from build123d import *

# Parameters (mm, degrees)
F0_W     = 177.8
F0_H     = 127
F1_DEPTH = 76.2
F2_R     = 12.7
F4_DEPTH = 101.6
F6_DEPTH = 50.8
F8_DEPTH = 50.8
F9_R     = 5.08
F10_R    = 5.08


with BuildPart() as f1:
    # F0 (on Top) → F1 (new body)
    with BuildSketch(Plane.XY):
        with Locations((-8.271977, -2.472461)):
            Rectangle(F0_W, F0_H)
        with BuildLine():
            Line((-83.807927, -45.345337), (-83.807927, 28.44747))
            ThreePointArc((-83.807927, 28.44747), (-70.589135, 37.835685), (-57.370342, 28.44747))
            Line((-57.370342, 28.44747), (-57.370342, -45.345337))
            ThreePointArc((-57.370342, -45.345337), (-70.589135, -54.660871), (-83.807927, -45.345337))
        make_face(mode=Mode.SUBTRACT)
        with BuildLine():
            ThreePointArc((38.502203, 28.44747), (51.139944, 41.085211), (63.777684, 28.44747))
            Line((63.777684, 28.44747), (63.777684, -45.345337))
            ThreePointArc((63.777684, -45.345337), (51.139944, -57.983078), (38.502203, -45.345337))
            Line((38.502203, -45.345337), (38.502203, 28.44747))
        make_face(mode=Mode.SUBTRACT)
    extrude(amount=F1_DEPTH)

    # F2
    f2_edges = [f1.edges().sort_by_distance(p)[0] for p in [
        (80.628023, 61.027539, 38.1),
        (80.628023, -65.972461, 38.1),
        (-97.171977, 61.027539, 38.1),
        (-97.171977, -65.972461, 38.1),
    ]]
    fillet(f2_edges, radius=F2_R)

    # F3 (on face) → F4 (join)
    with BuildSketch(Plane.XY.offset(76.2)):
        with BuildLine():
            ThreePointArc((0.43315, 40.995162), (-7.205375, 48.633687), (-14.8439, 40.995162))
            Line((-14.8439, 40.995162), (-14.8439, 15.583021))
            Line((-14.8439, 15.583021), (-41.930374, 15.583021))
            ThreePointArc((-41.930374, 15.583021), (-49.721884, 7.79151), (-41.930374, 0))
            Line((-41.930374, 0), (-14.8439, 0))
            Line((-14.8439, 0), (-14.8439, -28.666684))
            ThreePointArc((-14.8439, -28.666684), (-7.42195, -36.088634), (0, -28.666684))
            Line((0, -28.666684), (0, 0))
            Line((0, 0), (25.956901, 0))
            ThreePointArc((25.956901, 0), (33.748411, 7.79151), (25.956901, 15.583021))
            Line((25.956901, 15.583021), (0.43315, 15.583021))
            Line((0.43315, 15.583021), (0.43315, 40.995162))
        make_face()
    extrude(amount=F4_DEPTH)

    # F5 (on face) → F6 (join)
    with BuildSketch(Plane.YZ):
        Polygon((-16.809505, 118.773863), (-10.288356, 118.773863), (-7.027781, 124.421343), (-10.288356, 130.068824), (-16.809505, 130.068824), (-20.070079, 124.421343), align=None)
    extrude(amount=F6_DEPTH)

    # F7 (on face) → F8 (join)
    with BuildSketch(Plane(origin=(-14.8439, 0, 0), x_dir=(0, -1, 0), z_dir=(-1, 0, 0))):
        Polygon((15.825561, 128.772154), (10.70182, 128.772154), (8.139949, 124.334864), (10.70182, 119.897574), (15.825561, 119.897574), (18.387432, 124.334864), align=None)
    extrude(amount=F8_DEPTH)

    # F9
    f9_edges = [f1.edges().sort_by_distance(p)[0] for p in [
        (0.43315, 28.289091, 177.8),
        (-7.205375, 48.633687, 177.8),
        (-14.8439, 28.289091, 177.8),
        (-28.387137, 15.583021, 177.8),
        (-49.721884, 7.79151, 177.8),
        (-28.387137, 0, 177.8),
        (-14.8439, -14.333342, 177.8),
        (-7.42195, -36.088634, 177.8),
        (0, -14.333342, 177.8),
        (12.97845, 0, 177.8),
        (33.748411, 7.79151, 177.8),
        (13.195026, 15.583021, 177.8),
    ]]
    fillet(f9_edges, radius=F9_R)

    # F10
    f10_edges = [f1.edges().sort_by_distance(p)[0] for p in [
        (-97.171977, -2.472461, 0),
        (-97.171977, 48.327539, 38.1),
        (-97.171977, -53.272461, 38.1),
        (-97.171977, -2.472461, 76.2),
    ]]
    fillet(f10_edges, radius=F10_R)


solid = f1.part
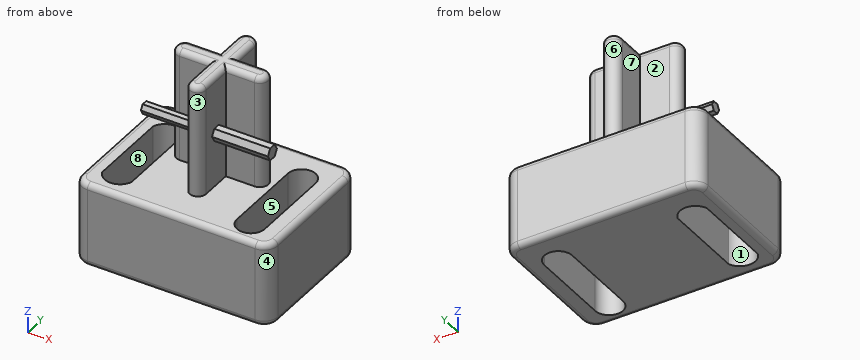
Here's how the part is built. I have some questions about the finished solid (model axes, mm). Face numbers are marked on the shaded views. A direction names the side the tool comes from. Round coordinates to 2 decimals unless told otherwise and drop trailing zeros. Order: outer loops, then holes, each group sorted by start corner. A loop starts at its lowest first (then second) coordinate and runs counter-clockwise, first axis right, second up. Notation, with made-up numbers: M 54.25,55.5 L 106.25,55.5 A29 cw 106.25,90.5 Z; hole C 32,-2.5 d7. An arc over 180 degrees is marked long. Return JSON: item names as keys, results as strings. Group by question number.
1. If we section it at C-C on z = 47: List the corners of the cut face in (x, y) for me, then the cut area to 3 significant figures.
2. If we mould it in two halves opening along X, with no side actions, what happens to the marked faces 1, 2, 3 and 4? For each: pulls with the +X half, pulls with the -X half, needs draft (parallel to the pull), parting line crosses it, or undercut.
3. Please list where these lines run through material, in increasing order: probe 1 along X at (y, z) = (24.5, 17); probe 2 along X at (y, z) = (34.5, 41.5); probe 3 along Z at (x, y) = (-42.5, -35).
4. If we section it at A-A on y = -43: List the corners of the cut face in (x, z) for me.
5. If we section it at B-B on x = -28: List the corners of the cut face in (y, z) for me, then the cut area to 3 significant figures.
6. If we section it at D-D on z = 156.5: List the corners of the cut face in (x, y) for me, then the cut area to 3 significant figures.
7. On a 3-axis mill with a long thin cutter (end or side, diameter ignored), from which of +Z, -Z, +X, -X, +Y, -Y can I reach the whole of each face in a straight line? I mean the marked faces 5, 6, 7 and 8. Say none if no direction works.
8. I'm going to push flat-ended pins straight in: pin 1 Ø6 at (x, z) = (-26.5, 106.5) entering from +Y; pin 2 Ø1.5 at (x, y) = (-58, -16) entering from +Z; pin 3 Ø5 at (x, y) = (32, -12.5) entering from +Z. Where does each tip first touch, or does it pass through?
Reply:
{
 "1": {"outline": "M -97.17,-53.27 A12.7 ccw -84.47,-65.97 L 67.93,-65.97 A12.7 ccw 80.63,-53.27 L 80.63,48.33 A12.7 ccw 67.93,61.03 L -84.47,61.03 A12.7 ccw -97.17,48.33 Z; hole M -83.81,-45.35 A14.04 ccw -57.37,-45.35 L -57.37,28.45 A14 ccw -83.81,28.45 Z; hole M 38.5,-45.35 A12.64 ccw 63.78,-45.35 L 63.78,28.45 A12.64 ccw 38.5,28.45 Z", "area": "17,800 mm^2"},
 "2": {"face 1": "undercut", "face 2": "needs draft", "face 3": "parting line crosses it", "face 4": "pulls with the +X half"},
 "3": {"probe 1": "-97.17 to -83.81, -57.37 to 38.5, 63.78 to 80.63", "probe 2": "-97.17 to -79.66, -61.52 to 40.05, 62.23 to 80.63", "probe 3": "0 to 76.2"},
 "4": {"outline": "M -97.17,5.08 A5.08 ccw -92.09,0 L -83.81,0 L -83.81,76.2 L -92.09,76.2 A5.08 ccw -97.17,71.12 Z; M -57.37,0 L 38.5,0 L 38.5,76.2 L -57.37,76.2 Z; M 63.78,0 L 75.55,0 A5.08 ccw 80.63,5.08 L 80.63,71.12 A5.08 ccw 75.55,76.2 L 63.78,76.2 Z"},
 "5": {"outline": "M -65.97,5.08 A5.08 ccw -60.89,0 L 55.95,0 A5.08 ccw 61.03,5.08 L 61.03,71.12 A5.08 ccw 55.95,76.2 L 15.58,76.2 L 15.58,172.72 A5.08 ccw 10.5,177.8 L 5.08,177.8 A5.08 ccw 0,172.72 L 0,76.2 L -60.89,76.2 A5.08 ccw -65.97,71.12 Z; M -18.39,124.33 L -15.83,119.9 L -10.7,119.9 L -8.14,124.33 L -10.7,128.77 L -15.83,128.77 Z", "area": "11,300 mm^2"},
 "6": {"outline": "M -41.93,0 L -14.84,0 L -14.84,-28.67 A7.42 ccw 0,-28.67 L 0,0 L 25.96,0 A7.79 ccw 25.96,15.58 L 0.43,15.58 L 0.43,41 A7.64 ccw -14.84,41 L -14.84,15.58 L -41.93,15.58 A7.79 ccw Z", "area": "2,240 mm^2"},
 "7": {"face 5": "-Z", "face 6": "+Z, +Y", "face 7": "+Z, -X, +Y", "face 8": "+Z, -Z"},
 "8": {"pin 1": "y = 15.58", "pin 2": "z = 128.77", "pin 3": "z = 130.07"}
}
